from build123d import *

# Parameters (mm, degrees)
SKETCH1_R               = 12.5
BOSS_EXTRUDE1_DEPTH     = 3.3
CUT_EXTRUDE1_START      = -6.6
CUT_EXTRUDE1_DEPTH      = 26.469552194
CIRPATTERN2_COUNT       = 39
SKETCH2_R               = 15
BOSS_EXTRUDE3_DEPTH     = 1.5
BOSS_EXTRUDE4_START     = 1.5
SKETCH3_R               = 14.999999972
BOSS_EXTRUDE4_DEPTH     = 1.5
CUT_EXTRUDE2_DEPTH      = 24.284329494
CUT_EXTRUDE2_DEPTH_BACK = 24.284329494


with BuildPart() as part:
    # Sketch1 → Boss-Extrude1 (new, symmetric)
    with BuildSketch(Plane.XY):
        Circle(SKETCH1_R)
    extrude(amount=BOSS_EXTRUDE1_DEPTH, both=True)

    # Sketch4 → Cut-Extrude1 (cut)
    with BuildSketch(Plane.XY.offset(3.3).offset(CUT_EXTRUDE1_START)):
        Polygon((-0.6, 11.75), (0.6, 11.75), (0.8, 12.5), (-0.8, 12.5), align=None)
    cut_extrude1 = extrude(amount=CUT_EXTRUDE1_DEPTH, mode=Mode.SUBTRACT)

    # CirPattern2: Cut-Extrude1 ×39 about axis
    cirpattern2_axis = Axis((0, 0, 0), (0, 0, 1))
    for i in range(1, CIRPATTERN2_COUNT):
        add(cut_extrude1.rotate(cirpattern2_axis, i * 360 / CIRPATTERN2_COUNT), mode=Mode.SUBTRACT)

    # Sketch2 → Boss-Extrude3 (add)
    with BuildSketch(Plane(origin=(0, 0, -3.3), x_dir=(-1, 0, 0), z_dir=(0, 0, -1))):
        Circle(SKETCH2_R)
    extrude(amount=BOSS_EXTRUDE3_DEPTH)

    # Sketch3 → Boss-Extrude4 (add)
    with BuildSketch(Plane.XY.offset(3.3).offset(BOSS_EXTRUDE4_START)):
        with Locations(Location((0, 0, 0), (0, 0, 180))):
            Circle(SKETCH3_R)
    extrude(amount=-BOSS_EXTRUDE4_DEPTH)

    # Sketch5 → Cut-Extrude2 (cut, two sides: drawn at the far end of the back side and taken through both)
    with BuildSketch(Plane.XY.offset(4.8).offset(-CUT_EXTRUDE2_DEPTH_BACK)):
        Polygon((7.625, 0), (3.8125, 6.603443704), (-3.8125, 6.603443704), (-7.625, 0), (-3.8125, -6.603443704), (3.8125, -6.603443704), align=None)
    extrude(amount=CUT_EXTRUDE2_DEPTH + CUT_EXTRUDE2_DEPTH_BACK, mode=Mode.SUBTRACT)


solid = part.part
The model under review builds one solid part; all positions refer to its coordinate system, in mm. A direction names the side the tool comes from. Round coordinates to 2 decimals unless told otherwise and drop trailing zeros. Loops run counter-clockwise (first coordinate to the right, second up) from the corner with the lowest first, then second, coordinate; pieces in that order, holes last. Notation, with made-up numbers: (62.25, 69.5) -> (114.25, 69.5) arc R28 ccw to (114.25, 102.5) -> close; hole circle Ø7 at (78, 10). An arc over 180 degrees is marked (long way). One line per question, with ' | ' between items. Start each with the question number.
Item 1: For pin 1 (3 mm diameter, centred on x = -12, z = 3, fed in from -Y); pin 2 (1 mm diameter, centred on x = 0, z = 0.5, fed in from +Y); pin 3 (5 mm diameter, centred on y = -12, z = -3.5, fed in from +X), all flat-tipped, find the tip position at first contact; note any pin that passes through.
Item 2: Draft analysis for pull direction X (two halves, no side actions). For faces 1 (the face through (-6.92, 13.31, 4.06)), 2 (the face through (5.69, -3.35, -0.07)), 3 (the face through (-11.74, -0.48, -0.05)), state which applies: +X half, -X half, draft (parallel to the pull), parting line (faces both ways), or undercut.
Item 3: Add section B-B, the plane y = 5. Write out the cut boundary in (x, z).
Item 4: Wall thickness on line 1 along Z through (x, y) = (10.5, -10.25); line 2 along X through (y, z) = (9.25, -0.5); line 3 along X through (y, z) = (6.5, 0.25): over which ranges is each line inside the solid? List them lowest first. Write a range as [from, to].
Item 5: Machinability: for faces 4 (the face through (-5.745, -3.255, -0.067)), 5 (the face through (0, 11.75, 0)), 6 (the face through (-11.51, -2.36, -0.05)), 7 (the face through (9.11, -7.42, -0.05)), which of the approach directions +Z, -Z, +X, -X, +Y, -Y give a long, thin tool a straight path to every point of the face, cutting with its end or side? Answer none if there is none.
Item 6: Add section A-A, the plane z = 4.25. Write out the cut boundary in (x, y) (1 decimal).
Return value:
1) pin 1: stops at y = -10.68 | pin 2: stops at y = 11.75 | pin 3: stops at x = 11.61
2) face 1: parting line | face 2: undercut | face 3: -X half
3) outline: (-14.14, -4.8) -> (-4.74, -4.8) -> (-4.74, 4.8) -> (-14.14, 4.8) -> (-14.14, 3.3) -> (-10.63, 3.3) -> (-10.63, -3.3) -> (-14.14, -3.3) -> close; (4.74, -4.8) -> (14.14, -4.8) -> (14.14, -3.3) -> (10.63, -3.3) -> (10.63, 3.3) -> (14.14, 3.3) -> (14.14, 4.8) -> (4.74, 4.8) -> close
4) line 1: z = [-4.8, -3.3], [3.3, 4.8] | line 2: x = [-8.41, -7.81], [-7.25, 7.25], [7.81, 8.41] | line 3: x = [-9.79, -3.87], [3.87, 9.79]
5) face 4: +Z, -Z | face 5: +Y | face 6: -X | face 7: none
6) outline: circle Ø30 at (0, 0); hole (-7.6, 0) -> (-3.8, -6.6) -> (3.8, -6.6) -> (7.6, 0) -> (3.8, 6.6) -> (-3.8, 6.6) -> close
